```python
from build123d import *

# Parameters (mm, degrees)
BASE_FLANGE1_DEPTH           = 311.15
EDGE_FLANGE1_DEPTH           = 35.433
EDGE_FLANGE1_BEND_DEPTH      = 35.433
F_1_4_0_25_DIAMETER_HOLE1_D  = 6.35
F_10_0_1935_DIAMETER_HOLE1_D = 4.9149
FILLET1_R                    = 3.175
F_10_0_1935_DIAMETER_HOLE2_D = 4.9149
FILLET2_R                    = 1.524
F_1_4_0_25_DIAMETER_HOLE2_D  = 6.35
F_1_4_0_25_DIAMETER_HOLE3_D  = 6.35


# Sheet-metal steps are written as plain solids
with BuildPart() as part:
    # Sketch1 → Base-Flange1 (new, symmetric)
    with BuildSketch(Plane(origin=(0, 0, 0), x_dir=(0, 0, -1), z_dir=(1, 0, 0))):
        with BuildLine():
            Line((0, 0), (60.325, 0))
            ThreePointArc((60.325, 0), (62.57006403, 0.92993597), (63.5, 3.175))
            Line((63.5, 3.175), (63.5, 41.275))
            Line((63.5, 41.275), (66.675, 41.275))
            Line((66.675, 41.275), (66.675, 3.175))
            ThreePointArc((66.675, 3.175), (64.815128061, -1.315128061), (60.325, -3.175))
            Line((60.325, -3.175), (0, -3.175))
            Line((0, -3.175), (0, 0))
        make_face()
    extrude(amount=BASE_FLANGE1_DEPTH, both=True)

    # Edge-Flange1 section (across the edge) → Edge-Flange1 (add)
    with BuildSketch(Plane(origin=(-318.77, 41.275, -63.5), x_dir=(1, 0, 0), z_dir=(0, -1, 0))):
        with BuildLine():
            Line((0, 3.175), (0, 50.8))
            Line((0, 50.8), (3.175, 50.8))
            Line((3.175, 50.8), (3.175, 3.175))
            ThreePointArc((3.175, 3.175), (4.10493597, 0.92993597), (6.35, 0))
            Line((6.35, 0), (7.62, 0))
            Line((7.62, 0), (7.62, -3.175))
            Line((7.62, -3.175), (6.35, -3.175))
            ThreePointArc((6.35, -3.175), (1.859871939, -1.315128061), (0, 3.175))
        make_face()
    extrude(amount=EDGE_FLANGE1_DEPTH)

    # Edge-Flange1 section 2 (across the edge) → Edge-Flange1 bend (add)
    with BuildSketch(Plane(origin=(318.77, 5.842, -63.5), x_dir=(-1, 0, 0), z_dir=(0, 1, 0))):
        with BuildLine():
            Line((0, 3.175), (0, 50.8))
            Line((0, 50.8), (3.175, 50.8))
            Line((3.175, 50.8), (3.175, 3.175))
            ThreePointArc((3.175, 3.175), (4.10493597, 0.92993597), (6.35, 0))
            Line((6.35, 0), (7.62, 0))
            Line((7.62, 0), (7.62, -3.175))
            Line((7.62, -3.175), (6.35, -3.175))
            ThreePointArc((6.35, -3.175), (1.859871939, -1.315128061), (0, 3.175))
        make_face()
    extrude(amount=EDGE_FLANGE1_BEND_DEPTH)

    # 1/4 (0.25) Diameter Hole1 (through all)
    with Locations(Plane(origin=(0, 0, 0), x_dir=(1, 0, 0), z_dir=(0, 1, 0))):
        with Locations((-6.35, 9.525), (6.35, 9.525), (222.25, 9.525), (234.95, 9.525), (-222.25, 9.525), (-234.95, 9.525)):
            Hole(F_1_4_0_25_DIAMETER_HOLE1_D / 2)

    # #10 (0.1935) Diameter Hole1 (through all)
    with Locations(Plane(origin=(0, 0, 0), x_dir=(1, 0, 0), z_dir=(0, 1, 0))):
        with Locations((-293.37, 19.05), (-293.37, 35.56), (293.37, 19.05), (293.37, 35.56)):
            Hole(F_10_0_1935_DIAMETER_HOLE1_D / 2)

    # Fillet1
    fillet1_edges = [part.edges().sort_by_distance(p)[0] for p in [
        (311.15, -1.5875, 0),
        (-317.1825, 41.275, -12.7),
        (-317.1825, 5.842, -12.7),
        (317.1825, 5.842, -12.7),
        (317.1825, 41.275, -12.7),
        (-311.15, -1.5875, 0),
    ]]
    fillet(fillet1_edges, radius=FILLET1_R)

    # #10 (0.1935) Diameter Hole2 (through all)
    with Locations(Plane(origin=(318.77, 0, 0), x_dir=(0, 0, -1), z_dir=(1, 0, 0))):
        with Locations((25.4, 28.575)):
            Hole(F_10_0_1935_DIAMETER_HOLE2_D / 2)

    # Fillet2
    fillet2_edges = [part.edges().sort_by_distance(p)[0] for p in [
        (311.15, 5.842, -65.0875),
        (-311.15, 5.842, -65.0875),
    ]]
    fillet(fillet2_edges, radius=FILLET2_R)

    # 1/4 (0.25) Diameter Hole2 (through all)
    with Locations(Plane.XY.offset(-63.5)):
        with Locations((-38.1, 7.9375), (38.1, 7.9375), (114.3, 7.9375), (190.5, 7.9375), (266.7, 7.9375), (-114.3, 7.9375), (-190.5, 7.9375), (-266.7, 7.9375)):
            Hole(F_1_4_0_25_DIAMETER_HOLE2_D / 2)

    # 1/4 (0.25) Diameter Hole3 (through all)
    with Locations(Plane(origin=(0, 0, 0), x_dir=(1, 0, 0), z_dir=(0, 1, 0))):
        with Locations((-266.7, 53.975), (-190.5, 53.975), (-114.3, 53.975), (-38.1, 53.975), (38.1, 53.975), (114.3, 53.975), (190.5, 53.975), (266.7, 53.975)):
            Hole(F_1_4_0_25_DIAMETER_HOLE3_D / 2)


solid = part.part
```
Build history of the part. All positions in model axes, mm. A direction names the side the tool comes from. Round coordinates to 2 decimals unless told otherwise and drop trailing zeros. Write each loop counter-clockwise with the first axis right and the second up, starting at its lowest first coordinate (ties: lowest second). Pieces come first, ordered by that corner, then holes.
1) Pin check, flat tips, straight feed: pin 1 (3 mm diameter, centred on x = 123.5, z = -21, fed in from +Y); pin 2 (12 mm diameter, centred on y = 11, z = -9, fed in from -X); pin 3 (3.5 mm diameter, centred on x = 317.5, y = 27.5, fed in from +Z); pin 4 (1.8 mm diameter, centred on x = -315.5, z = -37, fed in from -Y). Stop position of each tip, or through.
2) Band-saw the part on A-A, the plane x = -167. List the corners of the cut face in (y, z) (3 decimals).
3) Drill centre lines: probe 1 along X at (y, z) = (-1, -19.05); probe 2 along Z at (x, y) = (293.37, -2.1); probe 3 along Y at (x, z) = (32.5, -30.5) (3 decimals). Where is each one in solid material? Low to high.
4) 3-axis set-ups, long thin cutter, end or side, ignore diameter. For faces 5 (the flat face through (-315.595, 24, -36)), 6 (the flat face through (4, -3.175, -31)), 7 (the flat face through (4, 22, -63.5)): which of +Z, -Z, +X, -X, +Y, -Y reach the whole face in a straight line?
5) Mould opens along X. For faces 1 (the flat face through (318.77, 23, -37)), 2 (the flat face through (4, 0, -30)), 3 (the flat face through (-318.77, 24, -37)), 4 (the flat face through (315.595, 23, -36)) say: +X half, -X half, draft (parallel to the pull), parting line (faces both ways), or undercut.
Ans:
1. pin 1: stops at y = 0
1. pin 2: stops at x = -318.77
1. pin 3: stops at z = -12.7
1. pin 4: stops at y = 5.84
2. outline: (-3.175, -60.325) arc R6.35 ccw to (3.175, -66.675) - (41.275, -66.675) - (41.275, -63.5) - (3.175, -63.5) arc R3.175 cw to (0, -60.325) - (0, 0) - (-3.175, 0) - close
3. probe 1: x = -311.15 to -295.83, -290.91 to 290.91, 295.83 to 311.15
3. probe 2: z = -63.86 to -38.02, -33.1 to -21.51, -16.59 to 0
3. probe 3: y = -3.175 to 0
4. face 5: +Z, +Y, -Y
4. face 6: +Z, -Z, +X, -X, -Y
4. face 7: +Z, +Y
5. face 1: +X half
5. face 2: draft
5. face 3: -X half
5. face 4: undercut
